```python
from build123d import *

# Parameters (mm, degrees)
CROQUIS1_W              = 280
CROQUIS1_H              = 110
SALIENTE_EXTRUIR1_DEPTH = 12.7
CORTAR_EXTRUIR2_DEPTH   = 20
CROQUIS5_R              = 3.375
CORTAR_EXTRUIR5_DEPTH   = 30
CROQUIS6_R              = 3.375
CORTAR_EXTRUIR6_DEPTH   = 30


with BuildPart() as part:
    # Croquis1 → Saliente-Extruir1 (new body)
    with BuildSketch(Plane(origin=(0, 0, 0), x_dir=(1, 0, 0), z_dir=(0, 1, 0))):
        with Locations((14.294294294, 1.756756757)):
            Rectangle(CROQUIS1_W, CROQUIS1_H)
    extrude(amount=SALIENTE_EXTRUIR1_DEPTH)

    # Croquis2 → Cortar-Extruir2 (cut)
    with BuildSketch(Plane(origin=(0, 0, 0), x_dir=(1, 0, 0), z_dir=(0, 1, 0))):
        with BuildLine():
            Line((-100.705705706, -3.243243243), (129.294294294, -3.243243243))
            ThreePointArc((129.294294294, -3.243243243), (139.294294294, -13.243243243), (129.294294294, -23.243243243))
            Line((129.294294294, -23.243243243), (-100.705705706, -23.243243243))
            ThreePointArc((-100.705705706, -23.243243243), (-110.705705706, -13.243243243), (-100.705705706, -3.243243243))
        make_face()
    extrude(amount=CORTAR_EXTRUIR2_DEPTH, mode=Mode.SUBTRACT)

    # Croquis5 → Cortar-Extruir5 (cut)
    with BuildSketch(Plane.ZY.offset(125.705705706)):
        with Locations((38.243243243, 6.35)):
            Circle(CROQUIS5_R)
        with Locations((-41.756756757, 6.35)):
            Circle(CROQUIS5_R)
    extrude(amount=-CORTAR_EXTRUIR5_DEPTH, mode=Mode.SUBTRACT)

    # Croquis6 → Cortar-Extruir6 (cut)
    with BuildSketch(Plane(origin=(154.294294294, 0, 0), x_dir=(0, 0, -1), z_dir=(1, 0, 0))):
        with Locations((41.756756757, 6.35)):
            Circle(CROQUIS6_R)
        with Locations((-38.243243243, 6.35)):
            Circle(CROQUIS6_R)
    extrude(amount=-CORTAR_EXTRUIR6_DEPTH, mode=Mode.SUBTRACT)


solid = part.part
```
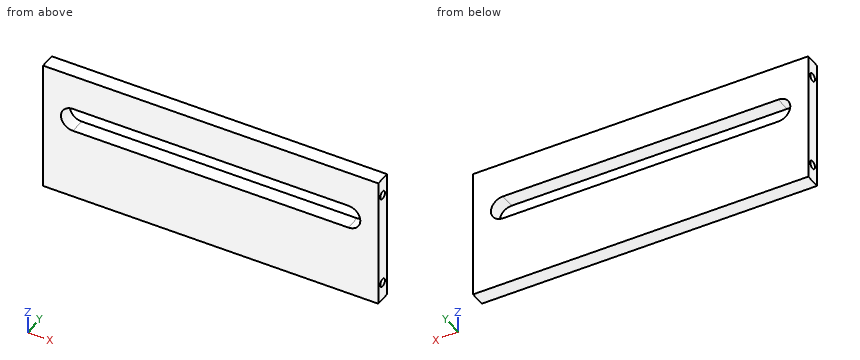
Geometry: final body of the model. Coordinates: model frame, mm. Coordinates: 2 decimals unless noted, no trailing zeros. Order: outer loops, then holes, each group sorted by start corner. A loop starts at its lowest first (then second) coordinate and runs counter-clockwise, first axis right, second up. Notation, with made-up numbers: M 56.5,85.5 L 113.5,85.5 A18 ccw 113.5,109.5 Z; hole C 50.5,-21 d6. An arc over 180 degrees is marked long. Answer in a Markdown table with one row per item. Add a question column.
Q1. Contact query for flat-ended pins moving along their axis: P1, Ø5.5, axis at y = 6.35, z = 38.24, coming from the +X side; P2, Ø2, axis at y = 6.5, z = -43.5, coming from the -X side. Output: stop coordinate, or through.
Q2. Section query B-B on y = 6.35. Return the cut outline in (x, z).
Q3. Line query: L1, parallel to Z at x = 65.5, y = 8.25; L2, parallel to Z at x = 137, y = 5.25; L3, parallel to Z at x = 136.5, y = 3.25. Output: solid intervals per line, ascending.
Q4. Section query A-A on x = 99. Return the cut outline in (y, z).
Completed:
| question | item | result |
|---|---|---|
| 1 | P1 | stops at x = 124.29 |
| 1 | P2 | stops at x = -95.71 |
| 2 | outline | M -125.71,-56.76 L 154.29,-56.76 L 154.29,-45.13 L 124.29,-45.13 L 124.29,-38.38 L 154.29,-38.38 L 154.29,34.87 L 124.29,34.87 L 124.29,41.62 L 154.29,41.62 L 154.29,53.24 L -125.71,53.24 L -125.71,41.62 L -95.71,41.62 L -95.71,34.87 L -125.71,34.87 L -125.71,-38.38 L -95.71,-38.38 L -95.71,-45.13 L -125.71,-45.13 Z; hole M -100.71,3.24 L 129.29,3.24 A10 ccw 129.29,23.24 L -100.71,23.24 A10 ccw Z |
| 3 | L1 | z = -56.76 to 3.24, 23.24 to 53.24 |
| 3 | L2 | z = -56.76 to -44.95, -38.57 to 6.87, 19.62 to 35.05, 41.43 to 53.24 |
| 3 | L3 | z = -56.76 to -43.09, -40.42 to 6.31, 20.18 to 36.91, 39.58 to 53.24 |
| 4 | outline | M 0,-56.76 L 12.7,-56.76 L 12.7,3.24 L 0,3.24 Z; M 0,23.24 L 12.7,23.24 L 12.7,53.24 L 0,53.24 Z |
